The drawing under review shows one solid part. Ordinate dimensions are in mm from its lowest x, y, z. A direction names the side the tool comes from. Give positions to 0.01 mm unless a question says otherwise; leave off trailing zeros. Loops run counter-clockwise (first coordinate to the right, second up) from the corner with the lowest first, then second, coordinate; pieces in that order, holes last. Notation, with made-up numbers: (81, -39.5) - (133, -39.5) arc R34 cw to (133, -7.5) - close; hole circle Ø8 at (-30.5, -25.75). An arc over 180 degrees is marked (long way). Write each question's results on one line, items separated by ' | '.
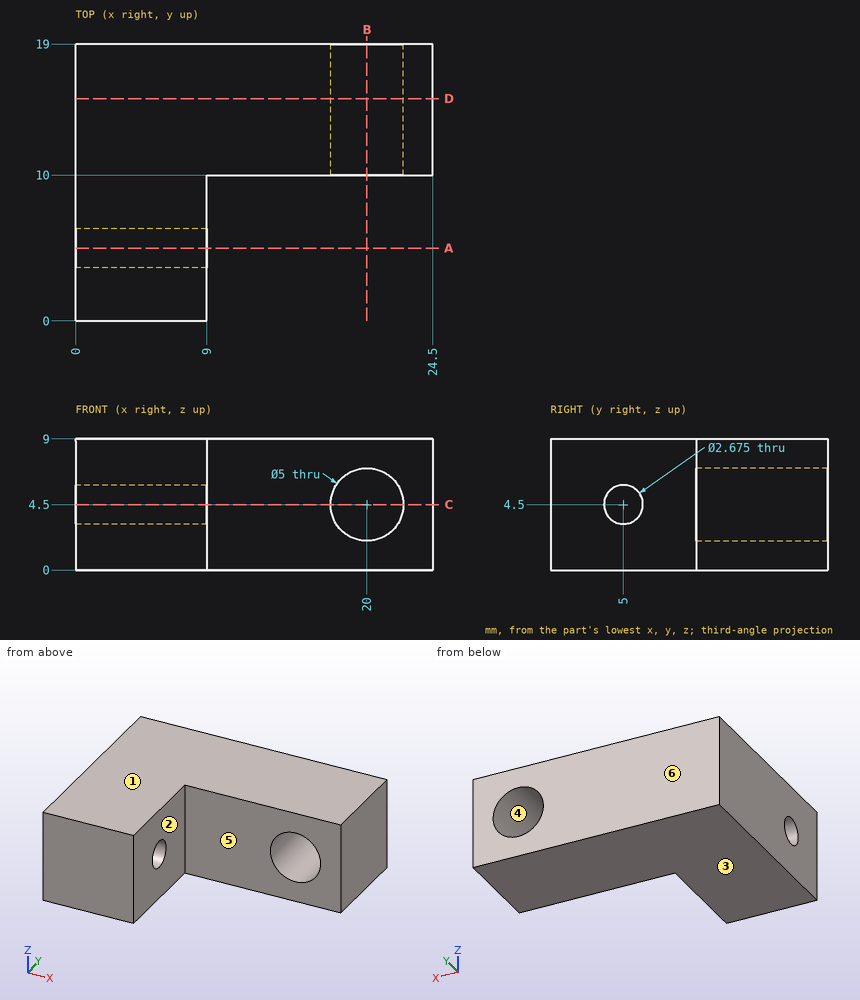
(1) Wall thickness on line 1 along X through (y, z) = (15.75, 4.5); line 2 along Z through (x, y) = (2.75, 5); line 3 along Z through (x, y) = (20, 12.5): over which ranges is each line inside the solid? List them lowest first. Write a range as from..to.
Answers below:
line 1: 0..17.5, 22.5..24.5 | line 2: 0..3.16, 5.84..9 | line 3: 0..2, 7..9
(2) Take a section at B-B on x = 20. Give the boundary of the cut face in (y, z), plus the area to 3 significant figures.
Answers below:
outline: (10, 0) - (19, 0) - (19, 2) - (10, 2) - close; (10, 7) - (19, 7) - (19, 9) - (10, 9) - close | area: 36.0 mm2
(3) Insertion check: P1, Ø3, axis at y = 3.5, z = 1, coming from the -X side. The pin has a flat end and moves straight along its axis. Give the tip position at first contact, or say it passes through.
Answers below:
P1: x = 0
(4) Take a section at D-D on y = 15.25. Give the boundary of the cut face in (x, z), plus the area to 3 significant figures.
Answers below:
outline: (0, 0) - (24.5, 0) - (24.5, 9) - (0, 9) - close; hole circle Ø5 at (20, 4.5) | area: 201 mm2
(5) Tool access review of the marked faces 5 and 6: name each direction out of +Z, -Z, +X, -X, +Y, -Y from which nothing blocks a thin tool from reaching the whole face with its end or side.
Answers below:
face 5: +Z, -Z, +X, -Y | face 6: +Z, -Z, +X, -X, +Y
(6) Take a section at A-A on y = 5. Give the boundary of the cut face in (x, z), plus the area to 3 significant figures.
Answers below:
outline: (0, 0) - (9, 0) - (9, 3.16) - (0, 3.16) - close; (0, 5.84) - (9, 5.84) - (9, 9) - (0, 9) - close | area: 56.9 mm2
(7) Take a section at C-C on z = 4.5. Give the boundary of the cut face in (x, y), plus the area to 3 significant figures.
Answers below:
outline: (0, 0) - (9, 0) - (9, 3.66) - (0, 3.66) - close; (0, 6.34) - (9, 6.34) - (9, 10) - (17.5, 10) - (17.5, 19) - (0, 19) - close; (22.5, 10) - (24.5, 10) - (24.5, 19) - (22.5, 19) - close | area: 241 mm2
(8) Draft analysis for pull direction Z (two halves, no side actions). For the marked faces 1, 2, 3 and 4, state which applies: pulls with the +Z half, pulls with the -Z half, needs draft (parallel to the pull), parting line crosses it, or undercut.
Answers below:
face 1: pulls with the +Z half | face 2: needs draft | face 3: pulls with the -Z half | face 4: undercut
